Autodesk Inventor part; units mm, degrees
ref_plane "YZ Plane" through (0, 0, 0) normal (1, 0, 0) x (0, 1, 0)
ref_plane "XZ Plane" through (0, 0, 0) normal (0, 1, 0) x (-1, 0, 0)
ref_plane "XY Plane" through (0, 0, 0) normal (0, 0, 1) x (1, 0, 0)
sketch "Boceto2" plane through (0, 0, 0) normal (0, 0, 1) x (1, 0, 0)
  line L0 (-81.2065, -59) -> (-81.2065, 59)
  line L1 (-81.2065, 59) -> (31.0181, 95.464)
  line L2 (31.0181, 95.464) -> (100.3768, 0)
  line L3 (100.3768, 0) -> (31.0181, -95.464)
  line L4 (31.0181, -95.464) -> (-81.2065, -59)
  line L5 (0, 0) -> (-162.4131, 0)
  line L6 (-162.4131, 0) -> (-162.4131, 162.4131)
  line L7 (-162.4131, 162.4131) -> (0, 162.4131)
  line L8 (0, 162.4131) -> (0, 0)
  line L9 (-162.4131, 162.4131) -> (-81.2065, 0)
  dimension "d3" = 118
  dimension "d4" = 262.7899
  dimension "d5" = 26.565
extrude "Extrusión1" add sketch "Boceto2" along normal blind 262.7899 draft 26.57 contours L0 L5 L8 L1 L2 L3 L4 | L0 L1 L8 L5
sketch "Boceto3" plane through (0, 0, 262.7899) normal (0, 0, 1) x (1, 0, 0)
  line L0 (-31.0181, 95.464) -> (81.2065, 59)
  line L1 (81.2065, 59) -> (81.2065, -59)
  line L2 (81.2065, -59) -> (-31.0181, -95.464)
  line L3 (-31.0181, -95.464) -> (-100.3768, 0)
  line L4 (-100.3768, 0) -> (-31.0181, 95.464)
  point P0 (0, 0)
  point P1 (0, 0)
  dimension "d8" = 118
extrude "Extrusión2" cut sketch "Boceto3" against normal blind 262.7899 draft 26.565 keep common part
ref_plane "Plano de trabajo1" through (-131.3998, -95.4675, 100.3648) normal (0.4910723, 0.3567849, 0.7947028) x (0.8506859, 0.0000184, -0.5256744)
feature "Dividir1" [suppressed]
ref_plane "Plano de trabajo2" through (31.0181, -95.464, 0) normal (-0.4910723, -0.3567849, -0.7947028) x (-0.8506859, -0.0000184, 0.5256744)
ref_plane "Plano de trabajo3" through (31.0181, -95.464, 0) normal (0.2628656, 0.809017, -0.5257311) x (-0.9510565, 0.309017, 0)
ref_plane "Plano de trabajo4" through (-81.2065, -59, 0) normal (-0.5877853, 0.809017, 0) x (-0.4253919, -0.3090653, 0.8506)
ref_plane "Plano de trabajo5" through (-81.2065, -59, 0) normal (0.8506508, 0, -0.5257311) x (0, 1, 0)
equation "\"d6\" = d4"
equation "\"d9\" = d4"
equation "\"d10\" = d5"
properties part number "Dodecaedro"
CAD build for the part. Positions are in the model's coordinates, mm. Coordinates: 2 decimals unless noted, no trailing zeros. Write each loop counter-clockwise with the first axis right and the second up, starting at its lowest first coordinate (ties: lowest second). Pieces come first, ordered by that corner, then holes. Notation, with made-up numbers: (-16, 51) -> (26, 51) arc R15 cw to (26, 73) -> close; hole circle Ø4 at (-35, 14.5). An arc over 180 degrees is marked (long way). Return JSON: item names as keys, results as strings. Group by question number.
Q1. Cut at A-A, the plane y = 68.5. Give the cut face in (x, z).
Q2. Flat gauge pins, fed straight in: pin 1 (4 mm diameter, centred on x = 83, z = 132.5, fed in from -Y); pin 2 (6 mm diameter, centred on x = -112, y = 98.5, fed in from +Z); pin 3 (5 mm diameter, centred on x = -27, z = 59, fed in from -Y). Where does each tip first touch, or does it go through?
Q3. Cut at D-D, the plane y = -82. Give the cut face in (x, z), then the cut area to 3 significant figures.
Q4. Cut at B-B, the plane z = 143.5. Give the cut face in (x, y), then the cut area to 3 significant figures.
Q5. Cut at C-C, the plane x = -126.5. Give the cut face in (y, z).
Q6. Drill centre lines: line 1 (Y direction, x = -128.5, z = 119); line 2 (Z direction, x = 77, y = 72.5); line 3 (Z direction, x = -44, y = 101). Where is each one in solid material? Low to high.
Returned:
{
 "1": {"outline": "(-140.16, 117.89) -> (-94.28, 26.15) -> (-51.97, 0) -> (50.61, 0) -> (140.16, 144.87) -> (94.28, 236.64) -> (51.97, 262.79) -> (-50.61, 262.79) -> close"},
 "2": {"pin 1": "stops at y = -128.15", "pin 2": "stops at z = 134.19", "pin 3": "stops at y = -109.18"},
 "3": {"outline": "(-135.78, 109.12) -> (-112.86, 63.3) -> (-10.42, 0) -> (40.8, 0) -> (135.78, 153.65) -> (112.86, 199.48) -> (10.42, 262.79) -> (-40.8, 262.79) -> close", "area": "46,300 mm2"},
 "4": {"outline": "(-152.97, -29.08) -> (-74.93, -136.5) -> (-19.61, -154.47) -> (106.66, -113.44) -> (140.85, -66.39) -> (140.85, 66.39) -> (106.66, 113.44) -> (-19.61, 154.47) -> (-74.93, 136.5) -> (-152.97, 29.08) -> close", "area": "69,000 mm2"},
 "5": {"outline": "(-99.03, 104.11) -> (-91.91, 90.57) -> (91.91, 90.57) -> (99.03, 104.11) -> (0, 220.52) -> close"},
 "6": {"line 1": "y = -83.61 to 83.61", "line 2": "z = 47.39 to 239.71", "line 3": "z = 56.88 to 235.28"}
}
